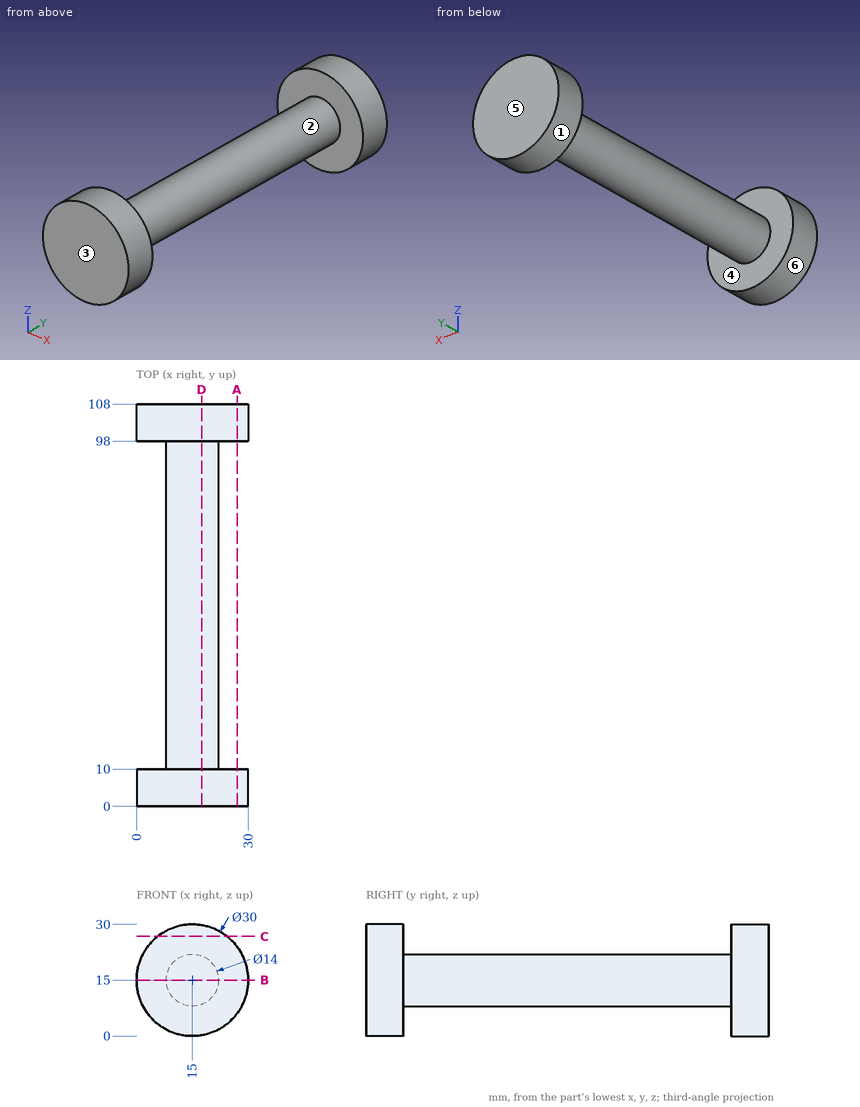
Verification items for this drawing (mm, ordinates from the low corner). A direction names the side the tool comes from. Coordinates: 2 decimals unless noted, no trailing zeros. Order: outer loops, then holes, each group sorted by start corner. A loop starts at its lowest first (then second) coordinate and runs counter-clockwise, first axis right, second up. Notation, with made-up numbers: (5.5, 55) -> (12.5, 55) arc R31 ccw to (12.5, 90) -> close; hole circle Ø11 at (52, 41.25). An arc over 180 degrees is marked (long way). Answer as CSV lines item,"result". Start each with the question number.
1) Cross-section at C-C, the plane z = 26.75. Record the boundary of the cut face in (x, y).
2) Cross-section at B-B, the plane z = 15. Record the boundary of the cut face in (x, y), then the cut area to 3 significant figures.
3) Cross-section at A-A, the plane x = 27. Record the boundary of the cut face in (y, z).
4) Gauge pin test, flat ends, axial feed: pin 1 Ø3 at (x, y) = (16.5, 41) entering from -Z; pin 2 Ø10 at (y, z) = (82, 9) entering from -X; pin 3 Ø8 at (y, z) = (47, 13) entering from +X; pin 4 Ø6 at (x, z) = (8.5, 23) entering from -Y. Record the tip position at first contact, or that the pin passes through.
5) Release check for a two-part mould opening along Y. For the marked faces 3, 4, 5 and 6 record: released by +Y, released by -Y, zero draft, split by the parting line, or undercut.
6) Material ranges on L1, parallel to Y at x = 10, z = 28.5; L2, parallel to X at y = 103, z = 28.5; L3, parallel to Z at x = 11.25, y = 58.5, recorded low to high. Write a range as [from, to].
7) Cross-section at D-D, the plane x = 17.5. Record the boundary of the cut face in (y, z), then the cut area to 3 significant figures.
8) Set-up check for the marked faces 1 and 2: record each of +Z, -Z, +X, -X, +Y, -Y from which the full face is reachable in a straight line by a thin tool's end or side.
Conclusion:
1,outline,"(5.68, 0) -> (24.32, 0) -> (24.32, 10) -> (5.68, 10) -> close; (5.68, 98) -> (24.32, 98) -> (24.32, 108) -> (5.68, 108) -> close"
2,outline,"(0, 0) -> (30, 0) -> (30, 10) -> (22, 10) -> (22, 98) -> (30, 98) -> (30, 108) -> (0, 108) -> (0, 98) -> (8, 98) -> (8, 10) -> (0, 10) -> close"
2,area,"1,830 mm²"
3,outline,"(0, 6) -> (10, 6) -> (10, 24) -> (0, 24) -> close; (98, 6) -> (108, 6) -> (108, 24) -> (98, 24) -> close"
4,pin 1,"stops at z = 8"
4,pin 2,"stops at x = 8.07"
4,pin 3,"stops at x = 22"
4,pin 4,"stops at y = 0"
5,face 3,"released by -Y"
5,face 4,"undercut"
5,face 5,"released by +Y"
5,face 6,"zero draft"
6,L1,"y = [0, 10], [98, 108]"
6,L2,"x = [8.46, 21.54]"
6,L3,"z = [9.09, 20.91]"
7,outline,"(0, 0.21) -> (10, 0.21) -> (10, 8.46) -> (98, 8.46) -> (98, 0.21) -> (108, 0.21) -> (108, 29.79) -> (98, 29.79) -> (98, 21.54) -> (10, 21.54) -> (10, 29.79) -> (0, 29.79) -> close"
7,area,"1,740 mm²"
8,face 1,"+Y, -Y"
8,face 2,"none"
